Source: CAD feature listing. Evaluate the final solid. Frame: model axes, mm. A direction names the side the tool comes from. Round coordinates to 2 decimals unless told otherwise and drop trailing zeros. Order: outer loops, then holes, each group sorted by start corner. A loop starts at its lowest first (then second) coordinate and runs counter-clockwise, first axis right, second up. Notation, with made-up numbers: (60, 35.25) - (104, 35.25) arc R5 cw to (104, 39.25) - close; hole circle Ø3 at (-32, 84.25). An arc over 180 degrees is marked (long way). Put each result on its own line as item: value. Start each with the question number.
1) Section A-A on x = -41.5. Output: boundary loops of the cut face in (y, z), then the cut area to 4 significant figures.
2) Section D-D on x = 0. Output: boundary loops of the cut face in (y, z).
3) Line query: probe 1 along X at (y, z) = (54.5, 2.4); probe 2 along X at (y, z) = (58.5, 3.15); probe 3 along Y at (x, z) = (-3, 2.4). Output: solid intervals per line, ascending. Write a range as [from, to].
4) Contact query for flat-ended pins moving along their axis: P1, Ø1.5, axis at x = -37.5, z = 3.5, coming from the -Y side; P2, Ø5, axis at x = -25, y = -4, coming from the +Z side; P3, Ø10, axis at x = 7, y = 8.5, coming from the +Z side; P4, Ø2, axis at x = -12.5, z = 1, coming from the -Y side. Output: stop coordinate, or through.
5) Section B-B on y = 34. Output: boundary loops of the cut face in (x, z).
6) Access query for faces 4 (the face through (52, 39, 4)), 5 (the face through (-50, 39, 1)), 6 (the face through (42, 0, 2)). Directions: +Z, -Z, +X, -X, +Y, -Y. A direction counts if a zero-diameter tool reaches every point of the face in a straight line with its end or side. Return the directions, or none.
7) Mould query, pull axis X, two halves, no side actions, for faces 1 (the face through (50, 39, 1)), 2 (the face through (-0.241, -14.93, 4.334)), 3 (the face through (-55, 39, 2)). Classes: +X half, -X half, draft (parallel to the pull), parting line (faces both ways), or undercut.
8) Section C-C on x = 22. Output: boundary loops of the cut face in (y, z).
```python
from build123d import *

# Parameters (mm, degrees)
F0_W     = 100.0000001118
F0_H     = 59.5
F0_W_2   = 40
F0_H_2   = 10
F1_DEPTH = 5
F2_W     = 104
F2_H     = 74
F2_W_2   = 100.0000001118
F2_H_2   = 59.5
F3_DEPTH = 2.5
F4_R     = 1.85
F5_DEPTH = 10
F6_R     = 9.99999


# Not quite as in the source:
# - a fillet or chamfer is up to 0.001 mm smaller than in the source, because OpenCascade refuses the exact size


with BuildPart() as f1:
    # F0 (on Top) → F1 (new body)
    with BuildSketch(Plane.XY):
        Polygon((-55, 77), (-55, 0), (-20, 0), (20, 0), (55, 0), (55, 77), align=None)
        with Locations((5.59e-08, 39.75)):
            Rectangle(F0_W, F0_H, mode=Mode.SUBTRACT)
        with Locations((0, -5)):
            Rectangle(F0_W_2, F0_H_2)
    extrude(amount=F1_DEPTH)

    # F2 (on face) → F3 (cut)
    with BuildSketch(Plane.XY.offset(5)):
        with Locations((0, 40)):
            Rectangle(F2_W, F2_H)
        with Locations((5.59e-08, 39.75)):
            Rectangle(F2_W_2, F2_H_2, mode=Mode.SUBTRACT)
    extrude(amount=-F3_DEPTH, mode=Mode.SUBTRACT)

    # F4 (on face) → F5 (join)
    with BuildSketch(Plane.XZ.offset(10)):
        with Locations((0, 2.5)):
            Circle(F4_R)
    extrude(amount=F5_DEPTH)

    # F6 (radius 10 in the source; OpenCascade refuses exactly that, so slightly less here)
    f6_edges = [f1.edges().sort_by_distance(p)[0] for p in [
        (20, 0, 2.5),
        (-20, 0, 2.5),
    ]]
    fillet(f6_edges, radius=F6_R)


solid = f1.part
```
Answer sheet:
1. outline: (0, 0) - (10, 0) - (10, 2.5) - (3, 2.5) - (3, 5) - (0, 5) - close; (69.5, 0) - (77, 0) - (77, 2.5) - (69.5, 2.5) - close
1. area: 51.25 mm^2
2. outline: (-20, 0.65) - (-10, 0.65) - (-10, 0) - (10, 0) - (10, 2.5) - (3, 2.5) - (3, 5) - (-10, 5) - (-10, 4.35) - (-20, 4.35) - close; (69.5, 0) - (77, 0) - (77, 2.5) - (69.5, 2.5) - close
3. probe 1: [-55, -50], [50, 55]
3. probe 2: [-55, -52], [52, 55]
3. probe 3: [-10, 10], [69.5, 77]
4. P1: y = 0
4. P2: z = 5
4. P3: z = 2.5
4. P4: y = -10
5. outline: (-55, 0) - (-50, 0) - (-50, 2.5) - (-52, 2.5) - (-52, 5) - (-55, 5) - close; (50, 0) - (55, 0) - (55, 5) - (52, 5) - (52, 2.5) - (50, 2.5) - close
6. face 4: +Z, +Y
6. face 5: +Z, -Z
6. face 6: +Z, -Z, +X, -Y
7. face 1: undercut
7. face 2: parting line
7. face 3: -X half
8. outline: (-4, 0) - (10, 0) - (10, 2.5) - (3, 2.5) - (3, 5) - (-4, 5) - close; (69.5, 0) - (77, 0) - (77, 2.5) - (69.5, 2.5) - close
